Read the model definition and answer for the solid it produces. Units are mm, in the model's axes. Face numbers are marked on the shaded views. A direction names the side the tool comes from. Give positions to 0.01 mm unless a question says otherwise; leave off trailing zeros. Loops run counter-clockwise (first coordinate to the right, second up) from the corner with the lowest first, then second, coordinate; pieces in that order, holes last. Notation, with made-up numbers: (46, 87.5) -> (70, 87.5) arc R24 ccw to (70, 106.5) -> close; hole circle Ø8 at (65.25, -4). An arc over 180 degrees is marked (long way). Write each question's results on one line, items separated by ' | '. Start each with the question number.
Item 1: Section C-C on y = 22 is taken. Write down the section's boundary in (x, z).
Item 2: Which of the six approach directions +Z, -Z, +X, -X, +Y, -Y give full straight-line access (tool end or side, diameter ignored) to the marked faces 1 and 2?
Item 3: Section D-D on z = 2.5 is taken. Write down the section's boundary in (x, y).
Item 4: Section A-A on x = -17.5 is taken. Write down the section's boundary in (y, z).
Item 5: Each of these flat-tipped pins is pushed along its axis until it touches: P1, Ø6, axis at x = 7.5, y = -3, coming from the +Z side; P2, Ø5, axis at x = -13, z = 14, coming from the -Y side; P3, Ø1, axis at x = 39, z = 27, coming from the -Y side. Where does it stop, or does it pass through?
Item 6: Section B-B on z = 14 is taken. Write down the section's boundary in (x, y).
Item 7: Find the intervals of material crossed by line 1 (Y direction, x = -3.5, z = 12); line 2 (X direction, y = 13.5, z = 23); line 3 (Z direction, x = -17, y = -31), in increasing order.
Item 8: Determine the mould class of the marked faces 3, 4 and 5 for opening direction X: +X half, -X half, draft (parallel to the pull), parting line (faces both ways), or undercut.
```python
from build123d import *

# Parameters (mm, degrees)
SKETCH_218_W                = 79
SKETCH_218_H                = 64
SKETCH_218_W_2              = 75
SKETCH_218_H_2              = 60
EXTRUDE_371_DEPTH           = 30
SKETCH_3_W                  = 79
SKETCH_3_H                  = 64
SKETCH_3_W_2                = 75
SKETCH_3_H_2                = 60
EXTRUDE_416_DEPTH           = 2
CUT_EXTRUDE_START           = -32
SKETCH_3_2_R                = 7.5
CUT_EXTRUDE_880_DEPTH       = 2
CUT_EXTRUDE_START_2         = 32
SKETCH_3_3_R                = 3
CUT_EXTRUDE_941_DEPTH       = 2
CUT_EXTRUDE_1138_DEPTH      = 60.027535947
CUT_EXTRUDE_1138_DEPTH_BACK = 60.027535947
SKETCH_4_W                  = 2
SKETCH_4_H                  = 8
FILLET_1191_R               = 2


with BuildPart() as part:
    # Sketch 218 → Extrude 371 (new body)
    with BuildSketch(Plane.XY):
        Rectangle(SKETCH_218_W, SKETCH_218_H)
        Rectangle(SKETCH_218_W_2, SKETCH_218_H_2, mode=Mode.SUBTRACT)
    extrude(amount=EXTRUDE_371_DEPTH)

    # Sketch 3 → Extrude 416 (add)
    # profile 1 of 2: a face of its own
    with BuildSketch(Plane.XY):
        Rectangle(SKETCH_3_W, SKETCH_3_H)
        Rectangle(SKETCH_3_W_2, SKETCH_3_H_2, mode=Mode.SUBTRACT)
    # profile 2 of 2: a face of its own
    with BuildSketch(Plane.XY):
        Rectangle(SKETCH_3_W_2, SKETCH_3_H_2)
    extrude(amount=-EXTRUDE_416_DEPTH)

    # Sketch 3 2 → Cut-Extrude 880 (cut)
    with BuildSketch(Plane(origin=(0, 0, 0), x_dir=(1, 0, 0), z_dir=(0, 1, 0)).offset(CUT_EXTRUDE_START)):
        with Locations(Location((-17.5, -14, 0), (0, 0, 270))):
            Circle(SKETCH_3_2_R)
    extrude(amount=CUT_EXTRUDE_880_DEPTH, mode=Mode.SUBTRACT)

    # 草图3<3> → Cut-Extrude 941 (cut)
    with BuildSketch(Plane(origin=(0, 0, 0), x_dir=(1, 0, 0), z_dir=(0, 1, 0)).offset(CUT_EXTRUDE_START_2)):
        with Locations(Location((17.5, -14, 0), (0, 0, 90))):
            Circle(SKETCH_3_3_R)
    extrude(amount=-CUT_EXTRUDE_941_DEPTH, mode=Mode.SUBTRACT)

    # 草图4 → Cut-Extrude 1138 (cut, two sides: drawn at the far end of the back side and taken through both)
    with BuildSketch(Plane(origin=(0, 0, 0), x_dir=(0, 0, -1), z_dir=(1, 0, 0)).offset(-CUT_EXTRUDE_1138_DEPTH_BACK)):
        with Locations((-27, 0)):
            Rectangle(SKETCH_4_W, SKETCH_4_H)
    extrude(amount=CUT_EXTRUDE_1138_DEPTH + CUT_EXTRUDE_1138_DEPTH_BACK, mode=Mode.SUBTRACT)

    # Fillet 1191
    fillet_1191_edges = [part.edges().sort_by_distance(p)[0] for p in [
        (-39.5, -32, 14),
        (-39.5, 32, 14),
        (39.5, 32, 14),
        (39.5, -32, 14),
    ]]
    fillet(fillet_1191_edges, radius=FILLET_1191_R)


solid = part.part
```
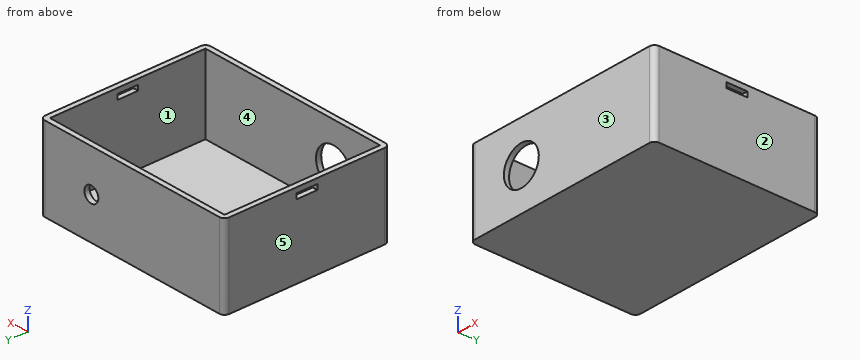
Findings:
1) outline: (-39.5, -2) -> (39.5, -2) -> (39.5, 30) -> (37.5, 30) -> (37.5, 0) -> (-37.5, 0) -> (-37.5, 30) -> (-39.5, 30) -> close
2) face 1: +Z | face 2: +Z, -Z, +X, +Y, -Y
3) outline: (-39.5, -30) arc R2 ccw to (-37.5, -32) -> (37.5, -32) arc R2 ccw to (39.5, -30) -> (39.5, 30) arc R2 ccw to (37.5, 32) -> (-37.5, 32) arc R2 ccw to (-39.5, 30) -> close; hole (-37.5, -30) -> (37.5, -30) -> (37.5, 30) -> (-37.5, 30) -> close
4) outline: (-32, -2) -> (32, -2) -> (32, 30) -> (30, 30) -> (30, 0) -> (-30, 0) -> (-30, 6.5) -> (-32, 6.5) -> close; (-32, 21.5) -> (-30, 21.5) -> (-30, 30) -> (-32, 30) -> close
5) P1: z = 0 | P2: y = 30 | P3: y = -31.73
6) outline: (-39.5, -30) arc R2 ccw to (-37.5, -32) -> (-25, -32) -> (-25, -30) -> (-37.5, -30) -> (-37.5, 30) -> (14.5, 30) -> (14.5, 32) -> (-37.5, 32) arc R2 ccw to (-39.5, 30) -> close; (-10, -32) -> (37.5, -32) arc R2 ccw to (39.5, -30) -> (39.5, 30) arc R2 ccw to (37.5, 32) -> (20.5, 32) -> (20.5, 30) -> (37.5, 30) -> (37.5, -30) -> (-10, -30) -> close
7) line 1: -32 to -30, 30 to 32 | line 2: -39.5 to -37.5, 37.5 to 39.5 | line 3: -2 to 6.52, 21.48 to 30
8) face 3: draft | face 4: undercut | face 5: -X half
